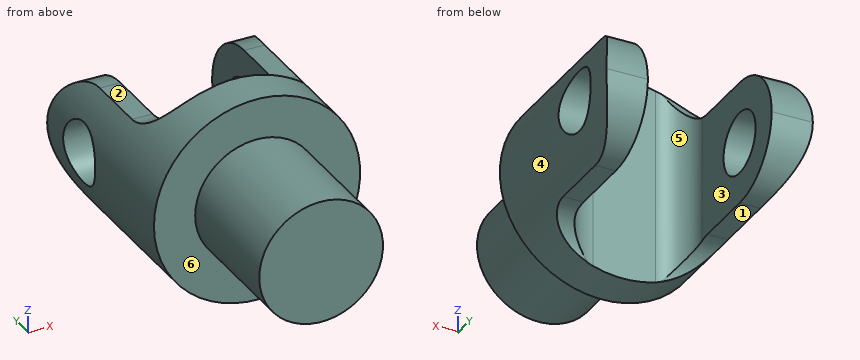
```python
from build123d import *

# Parameters (mm, degrees)
CORTAR_EXTRUIR1_DEPTH      = 5
CORTAR_EXTRUIR1_DEPTH_BACK = 5
CROQUIS2_R                 = 1.5
CORTAR_EXTRUIR2_DEPTH      = 5
CORTAR_EXTRUIR2_DEPTH_BACK = 5


with BuildPart() as part:
    # Croquis1 → Revoluci_n1 (revolve)
    with BuildSketch(Plane.XY, mode=Mode.PRIVATE) as revoluci_n1_sk:
        Polygon((3, 5), (5, 5), (5, -5), (3, -5), (3, -11), (0, -11), (0, -3), (0, 5), align=None)
    revolve(revoluci_n1_sk.sketch.rotate(Axis((0, -3, 0), (0, -1, 0)), 180), axis=Axis((0, -3, 0), (0, -1, 0)))

    # Croquis2 → Cortar-Extruir1 (cut, two sides: drawn at the far end of the back side and taken through both)
    with BuildSketch(Plane(origin=(0, 0, 0), x_dir=(0, 0, -1), z_dir=(1, 0, 0)).offset(-CORTAR_EXTRUIR1_DEPTH_BACK)):
        with BuildLine():
            Line((-5, 5), (-5, -3))
            Line((-5, -3), (-4.99, -3))
            ThreePointArc((-4.99, -3), (-3.582857505, -2.417142495), (-3, -1.01))
            Line((-3, -1.01), (-3, 2))
            ThreePointArc((-3, 2), (-2.121320344, 4.121320344), (0, 5))
            Line((0, 5), (-5, 5))
        make_face()
        with BuildLine():
            Line((5, 5), (0, 5))
            ThreePointArc((0, 5), (2.121320344, 4.121320344), (3, 2))
            Line((3, 2), (3, -1.01))
            ThreePointArc((3, -1.01), (3.582857505, -2.417142495), (4.99, -3))
            Line((4.99, -3), (5, -3))
            Line((5, -3), (5, 5))
        make_face()
        with Locations(Location((0, 2, 0), (0, 0, 90))):
            Circle(CROQUIS2_R)
    extrude(amount=CORTAR_EXTRUIR1_DEPTH + CORTAR_EXTRUIR1_DEPTH_BACK, mode=Mode.SUBTRACT)

    # Croquis3 → Cortar-Extruir2 (cut, two sides: drawn at the far end of the back side and taken through both)
    with BuildSketch(Plane.XY.offset(-CORTAR_EXTRUIR2_DEPTH_BACK)):
        with BuildLine():
            Line((3, -1.51), (3, 5))
            Line((3, 5), (-3, 5))
            Line((-3, 5), (-3, -1.51))
            ThreePointArc((-3, -1.51), (-2.563589104, -2.563589104), (-1.51, -3))
            Line((-1.51, -3), (1.51, -3))
            ThreePointArc((1.51, -3), (2.563589104, -2.563589104), (3, -1.51))
        make_face()
    extrude(amount=CORTAR_EXTRUIR2_DEPTH + CORTAR_EXTRUIR2_DEPTH_BACK, mode=Mode.SUBTRACT)


solid = part.part
```
The listing builds one solid part. Answer for the finished solid, in the listing's coordinates (mm). Face numbers are marked on the shaded views. A direction names the side the tool comes from. Coordinates: 2 decimals unless noted, no trailing zeros. Write each loop counter-clockwise with the first axis right and the second up, starting at its lowest first coordinate (ties: lowest second). Pieces come first, ordered by that corner, then holes.
Q1. Which of the six approach directions +Z, -Z, +X, -X, +Y, -Y give full straight-line access (tool end or side, diameter ignored) to the marked faces 1, 2 and 3?
Returned:
face 1: -Z, +X, -X, +Y
face 2: +Z, +X, -X, +Y
face 3: +Z, -Z, +Y
Q2. Section A-A, the plane y = 3.25 is taken. Write down the section's boundary in (x, z), then the cut area to 3 significant figures.
Returned:
outline: (-4.93, -0.83) arc R5 ccw to (-4.19, -2.73) - (-3, -2.73) - (-3, -0.83) - close; (-4.93, 0.83) - (-3, 0.83) - (-3, 2.73) - (-4.19, 2.73) arc R5 ccw to start; (3, -2.73) - (4.19, -2.73) arc R5 ccw to (4.93, -0.83) - (3, -0.83) - close; (3, 0.83) - (4.93, 0.83) arc R5 ccw to (4.19, 2.73) - (3, 2.73) - close
area: 12.4 mm2
Q3. Find the intervals of material crossed by line 1 along Z through (x, y) = (-3.45, 2); line 2 along Y through (x, z) = (1, -1); line 3 along X through (y, z) = (0.5, 0.75), in increasing order.
Returned:
line 1: z = -3 to -1.5, 1.5 to 3
line 2: y = -11 to -3
line 3: x = -4.94 to -3, 3 to 4.94
Q4. Section B-B, the plane x = 3.5 is taken. Write down the section's boundary in (y, z).
Returned:
outline: (-5, -3.57) - (-2.4, -3.57) arc R1.99 cw to (-1.01, -3) - (2, -3) arc R3 ccw to (2, 3) - (-1.01, 3) arc R1.99 cw to (-2.4, 3.57) - (-5, 3.57) - close; hole circle Ø3 at (2, 0)
Q5. Section D-D, the plane y = -4.5 is taken. Write down the section's boundary in (x, z).
Returned:
outline: circle Ø10 at (0, 0)
Q6. The mould has two halves that part along X. Classify the marked faces 4, 5 and 6: released by +X, released by -X, zero draft, split by the parting line, or undercut.
Returned:
face 4: split by the parting line
face 5: undercut
face 6: zero draft
Q7. Given P1, Ø5, axis at y = 2, z = 0, coming from the +X side; P2, Ø0.8, axis at x = 3.5, y = 1, coming from the -Z side; P3, Ø1.8, axis at y = 2, z = 0, coming from the -X side; P4, Ø2, axis at x = -3, y = -7, coming from the +Z side, each flat-ended and moving along its own axis, determine where each tip first touches the part or whether it passes through.
Returned:
P1: stops at x = 5
P2: stops at z = -3
P3: passes through
P4: stops at z = 2.24
Q8. Section C-C, the plane x = 0 is taken. Write down the section's boundary in (y, z), then the cut area to 3 significant figures.
Returned:
outline: (-11, -3) - (-5, -3) - (-5, -5) - (-3, -5) - (-3, 5) - (-5, 5) - (-5, 3) - (-11, 3) - close
area: 56.0 mm2
